Source: CAD feature listing. Evaluate the final solid. Frame: model axes, mm. Face numbers are marked on the shaded views. Coordinates: 2 decimals unless noted, no trailing zeros. Write each loop counter-clockwise with the first axis right and the second up, starting at its lowest first coordinate (ties: lowest second). Pieces come first, ordered by that corner, then holes. Notation, with made-up numbers: (71.5, 88) - (125.5, 88) arc R27 ccw to (125.5, 115) - close; hole circle Ø3 at (-12, 69.5). An arc over 180 degrees is marked (long way). One line per item, written item: value.
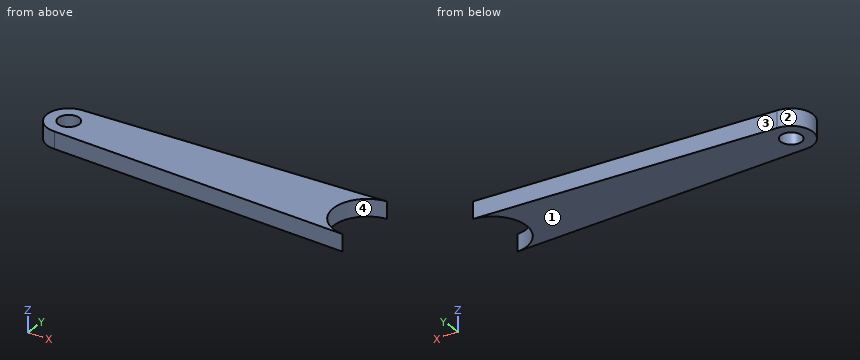
from build123d import *

# Parameters (mm, degrees)
SKETCH1_R           = 8.128
SKETCH1_R_2         = 3.937
BOSS_EXTRUDE1_DEPTH = 6.35
BOSS_EXTRUDE2_DEPTH = 6.35


with BuildPart() as part:
    # Sketch1 → Boss-Extrude1 (new body)
    with BuildSketch(Plane.XY):
        Circle(SKETCH1_R)
        Circle(SKETCH1_R_2, mode=Mode.SUBTRACT)
    extrude(amount=BOSS_EXTRUDE1_DEPTH)

    # Sketch2 → Boss-Extrude2 (add)
    with BuildSketch(Plane.XY.offset(6.35)):
        with BuildLine():
            Line((112.260554909, 12.658695041), (0, 8.128))
            ThreePointArc((0, 8.128), (5.747363917, 5.747363917), (8.128, 0))
            ThreePointArc((8.128, 0), (5.747363917, -5.747363917), (0, -8.128))
            Line((0, -8.128), (112.260554909, -12.658695041))
            ThreePointArc((112.260554909, -12.658695041), (100.584, 0), (112.260554909, 12.658695041))
        make_face()
    extrude(amount=-BOSS_EXTRUDE2_DEPTH)


solid = part.part
1) Section query A-A on y = 0. Output: boundary loops of the cut face in (x, z).
Values found:
outline: (-8.13, 0) - (-3.94, 0) - (-3.94, 6.35) - (-8.13, 6.35) - close; (3.94, 0) - (100.58, 0) - (100.58, 6.35) - (3.94, 6.35) - close
2) Draft query along Y for the marked faces 1, 2, 3 and 4. Return one class per face: released by +Y, released by -Y, zero draft, split by the parting line, or undercut.
Values found:
face 1: zero draft
face 2: split by the parting line
face 3: released by +Y
face 4: undercut
3) Section query D-D on y = -10. Output: boundary loops of the cut face in (x, z).
Values found:
outline: (46.38, 0) - (105.46, 0) - (105.46, 6.35) - (46.38, 6.35) - close
4) Contact query for flat-ended pins moving along their axis: P1, Ø1, axis at x = 85, z = 4.5, coming from the +Y side; P2, Ø1, axis at x = 16.5, z = 4, coming from the +Y side; P3, Ø4.5, axis at x = 0, y = 0, coming from the +Z side; P4, Ø1.5, axis at x = 62, z = 4, coming from the -Y side. Output: stop coordinate, or through.
Values found:
P1: y = 11.58
P2: y = 8.81
P3: through
P4: y = -10.66
5) Section query C-C on x = 96. Output: boundary loops of the cut face in (y, z), then the cut area to 3 significant figures.
Values found:
outline: (-12, 0) - (12, 0) - (12, 6.35) - (-12, 6.35) - close
area: 152 mm2
6) Section query B-B on z = 1.25. Output: boundary loops of the cut face in (x, y).
Values found:
outline: (0, -8.13) - (112.26, -12.66) arc R12.7 cw to (112.26, 12.66) - (0, 8.13) arc R8.13 ccw to start; hole circle Ø7.87 at (0, 0)
7) Material intervals for line 1 (X direction, y = 0.5, z = 6); line 2 (X direction, y = 1.5, z = 2.5); line 3 (Y direction, x = 103.5, z = 3.5), sorted ascending.
Values found:
line 1: -8.11 to -3.91, 3.91 to 100.59
line 2: -7.99 to -3.64, 3.64 to 100.67
line 3: -12.31 to -8.1, 8.1 to 12.31
